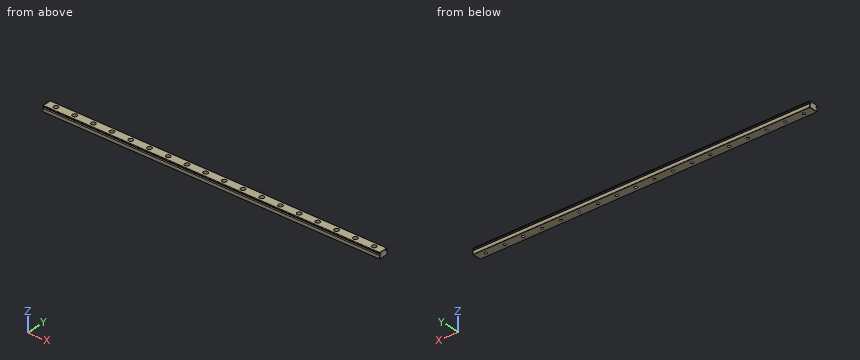
```python
from build123d import *

# Parameters (mm, degrees)
BOSS_EXTRUDE1_DEPTH   = 450
SKETCH2_R             = 1.75
CUT_EXTRUDE1_DEPTH    = 10
SKETCH3_R             = 3
CUT_EXTRUDE2_DEPTH    = 4
CHAMFER1_SIZE         = 0.5
CHAMFER1_SIZE2        = 1.743707222
CHAMFER1_PART_2_SIZE  = 0.5
CHAMFER1_PART_2_SIZE2 = 1.743707222
FILLET1_R             = 0.5


with BuildPart() as part:
    # Sketch1 → Boss-Extrude1 (new body)
    with BuildSketch(Plane(origin=(0, 0, 0), x_dir=(0, 0, -1), z_dir=(1, 0, 0))):
        Polygon((-0.5, 6), (4, 6), (4, -6), (-0.5, -6), (-0.5, -4.25), (-2.5, -4.25), (-2.5, -6), (-4, -6), (-4, 6), (-2.5, 6), (-2.5, 4.25), (-0.5, 4.25), align=None)
    extrude(amount=BOSS_EXTRUDE1_DEPTH)

    # Sketch2 → Cut-Extrude1 (cut)
    with BuildSketch(Plane.XY.offset(4)):
        with Locations((12.5, 0)):
            Circle(SKETCH2_R)
        with Locations((37.5, 0)):
            Circle(SKETCH2_R)
        with Locations((62.5, 0)):
            Circle(SKETCH2_R)
        with Locations((87.5, 0)):
            Circle(SKETCH2_R)
        with Locations((112.5, 0)):
            Circle(SKETCH2_R)
        with Locations((137.5, 0)):
            Circle(SKETCH2_R)
        with Locations((162.5, 0)):
            Circle(SKETCH2_R)
        with Locations((187.5, 0)):
            Circle(SKETCH2_R)
        with Locations((212.5, 0)):
            Circle(SKETCH2_R)
        with Locations((237.5, 0)):
            Circle(SKETCH2_R)
        with Locations((262.5, 0)):
            Circle(SKETCH2_R)
        with Locations((287.5, 0)):
            Circle(SKETCH2_R)
        with Locations((312.5, 0)):
            Circle(SKETCH2_R)
        with Locations((337.5, 0)):
            Circle(SKETCH2_R)
        with Locations((362.5, 0)):
            Circle(SKETCH2_R)
        with Locations((387.5, 0)):
            Circle(SKETCH2_R)
        with Locations((412.5, 0)):
            Circle(SKETCH2_R)
        with Locations((437.5, 0)):
            Circle(SKETCH2_R)
    extrude(amount=-CUT_EXTRUDE1_DEPTH, mode=Mode.SUBTRACT)

    # Sketch3 → Cut-Extrude2 (cut)
    with BuildSketch(Plane.XY.offset(4)):
        with Locations((12.5, 0)):
            Circle(SKETCH3_R)
        with Locations((37.5, 0)):
            Circle(SKETCH3_R)
        with Locations((62.5, 0)):
            Circle(SKETCH3_R)
        with Locations((87.5, 0)):
            Circle(SKETCH3_R)
        with Locations((112.5, 0)):
            Circle(SKETCH3_R)
        with Locations((137.5, 0)):
            Circle(SKETCH3_R)
        with Locations((162.5, 0)):
            Circle(SKETCH3_R)
        with Locations((187.5, 0)):
            Circle(SKETCH3_R)
        with Locations((212.5, 0)):
            Circle(SKETCH3_R)
        with Locations((237.5, 0)):
            Circle(SKETCH3_R)
        with Locations((262.5, 0)):
            Circle(SKETCH3_R)
        with Locations((287.5, 0)):
            Circle(SKETCH3_R)
        with Locations((312.5, 0)):
            Circle(SKETCH3_R)
        with Locations((337.5, 0)):
            Circle(SKETCH3_R)
        with Locations((362.5, 0)):
            Circle(SKETCH3_R)
        with Locations((387.5, 0)):
            Circle(SKETCH3_R)
        with Locations((412.5, 0)):
            Circle(SKETCH3_R)
        with Locations((437.5, 0)):
            Circle(SKETCH3_R)
    extrude(amount=-CUT_EXTRUDE2_DEPTH, mode=Mode.SUBTRACT)

    # Chamfer1
    chamfer1_edges = [part.edges().sort_by_distance(p)[0] for p in [
        (225, -4.25, 0.5),
        (225, -4.25, 2.5),
    ]]
    chamfer1_side = [part.faces().sort_by_distance(p)[0] for p in [
        (225, -4.25, 1.5),
    ]]
    chamfer(chamfer1_edges, length=CHAMFER1_SIZE, length2=CHAMFER1_SIZE2, reference=chamfer1_side[0])

    # Chamfer1 part 2
    chamfer1_part_2_edges = [part.edges().sort_by_distance(p)[0] for p in [
        (225, 4.25, 2.5),
        (225, 4.25, 0.5),
    ]]
    chamfer1_part_2_side = [part.faces().sort_by_distance(p)[0] for p in [
        (225, 4.25, 1.5),
    ]]
    chamfer(chamfer1_part_2_edges, length=CHAMFER1_PART_2_SIZE, length2=CHAMFER1_PART_2_SIZE2, reference=chamfer1_part_2_side[0])

    # Fillet1
    fillet1_edges = [part.edges().sort_by_distance(p)[0] for p in [
        (450, -6, -1.75),
        (450, 0, -4),
        (450, 6, -1.75),
        (450, 6, 3.25),
        (450, 0, 4),
        (450, -6, 3.25),
        (0, -6, 3.25),
        (0, -6, -1.75),
        (0, 0, -4),
        (0, 6, -1.75),
        (0, 6, 3.25),
        (0, 0, 4),
        (225, -4.25, 1),
        (225, -4.25, 2),
        (225, 4.25, 2),
        (225, 4.25, 1),
        (225, -6, 4),
        (225, 6, 4),
        (225, -6, -4),
        (225, 6, -4),
    ]]
    fillet(fillet1_edges, radius=FILLET1_R)


solid = part.part
```
Build history of the part. All positions in model axes, mm. Give positions to 0.01 mm unless a question says otherwise; leave off trailing zeros. One line per question, with ' | ' between items.
Q1. Drill centre lines: line 1 along Y through (x, z) = (112.5, -2.45); line 2 along Z through (x, y) = (140, -0.5); line 3 along X through (y, z) = (4.5, 3.75). Where is each one in solid material? Low to high. Write a range as [from, to].
Filled sheet:
line 1: y = [-6, -1.75], [1.75, 6] | line 2: z = [-4, 0] | line 3: x = [0.07, 449.93]
Q2. Cut at A-A, the plane z = -2.25. Count the separate pieces of the cut face and the enclosed holes in it, plus the area to 3 significant figures.
Filled sheet:
separate pieces: 1 | enclosed holes: 18 | area: 5,230 mm²
Q3. Drop flat-ended pins along their axis: pin 1 (3 mm diameter, centred on x = 263.5, y = 0.5, fed in from +Z); pin 2 (3 mm diameter, centred on x = 162.5, y = 0, fed in from +Z). Give the stop position or say it passes through.
Filled sheet:
pin 1: stops at z = 0 | pin 2: passes through
